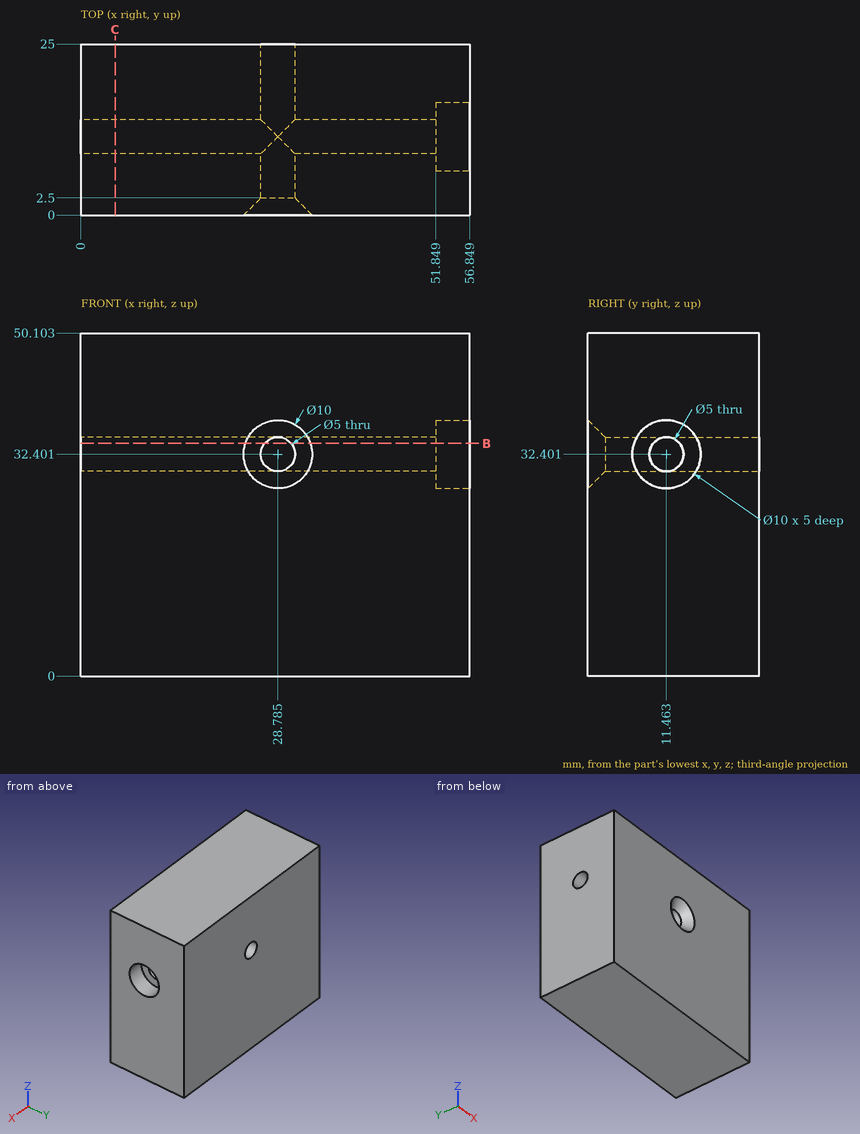
Check sheet for the drawn part. Datum: minimum x, y, z corner. Units: mm. Round coordinates to 2 decimals unless told otherwise and drop trailing zeros. Order: outer loops, then holes, each group sorted by start corner. A loop starts at its lowest first (then second) coordinate and runs counter-clockwise, first axis right, second up.
(1) Cross-section at C-C, the plane x = 5. Enter the section's corners in (y, z).
(2) Cross-section at B-B, the plane z = 34. State how many separate pieces and enclosed holes the cut face has, and give its area (3 significant figures).
(3) Go/stop test with flat-tipped pins: P1, Ø12, axis at x = 6, z = 9.5, coming from the -Y side; P2, Ø8, axis at y = 11.46, z = 32.4, coming from the +X side; P3, Ø4, axis at y = 11.46, z = 32.4, coming from the +X side. Record where each tip stops, or that it passes through.
(4) Scan lines: probe 1 along Z at (x, y) = (27.5, 15) (1 decimal); probe 2 along X at (y, z) = (11.5, 36); probe 3 along X at (y, z) = (3.5, 30.5). Record each from-to range of solid material in increasing order.
Check sheet entries:
1. outline: (0, 0) - (25, 0) - (25, 50.1) - (0, 50.1) - close; hole circle Ø5 at (11.46, 32.4)
2. separate pieces: 4
2. enclosed holes: 0
2. area: 1,090 mm2
3. P1: stops at y = 0
3. P2: stops at x = 51.85
3. P3: passes through
4. probe 1: z = 0 to 30.3, 34.5 to 50.1
4. probe 2: x = 0 to 51.85
4. probe 3: x = 0 to 27.16, 30.41 to 56.85
